Could you check a few things on this model? Use its own coordinates, in mm. A direction names the side the tool comes from. Give positions to 0.01 mm unless a question says otherwise; leave off trailing zeros. Order: outer loops, then holes, each group sorted by start corner. A loop starts at its lowest first (then second) coordinate and runs counter-clockwise, first axis right, second up. Notation, with made-up numbers: M 28,65 L 76,65 A26 ccw 76,83 Z; hole C -30.75,-19.75 d11. An arc over 180 degrees is marked long. Answer in a Markdown table with one row per item. Add a question column.
```python
from build123d import *

# Parameters (mm, degrees)
F0_W     = 101.6
F0_H     = 101.6
F1_DEPTH = 101.6
F2_R     = 76.2
F3_DEPTH = 152.4
F4_W     = 50.8
F4_H     = 50.8
F5_DEPTH = 50.8


with BuildPart() as f1:
    # F0 (on Front) → F1 (new body)
    with BuildSketch(Plane.XZ):
        with Locations((50.8, 50.8)):
            Rectangle(F0_W, F0_H)
    extrude(amount=-F1_DEPTH)

    # F2 (on face) → F3 (join)
    with BuildSketch(Plane.XY.offset(101.6)):
        Circle(F2_R)
    extrude(amount=F3_DEPTH)

    # F4 (on face) → F5 (join)
    with BuildSketch(Plane.XY.offset(101.6)):
        with Locations((76.2, 76.2)):
            Rectangle(F4_W, F4_H)
    extrude(amount=F5_DEPTH)


solid = f1.part
```
1. Suppose I cut it at C-C on z = 221. List the corners of the cut face in (x, y) for me.
2. For faces 1 (the flat face through (0, 50, 50)), 2 (the flat face through (79, 50.8, 127)), 3 (the flat face through (50, 0, 52)), which set-ups out of +Z, -Z, +X, -X, +Y, -Y let a thin tool reach every point of the face, with its end or its side?
3. If I drill on line 1 along Z through (x, y) = (34.5, 77); line 2 along Z through (x, y) = (-17, 28), over which ranges is the centre line in solid material (lowest first)? Write a range as [from, to].
4. Suppose I cut it at B-B on x = -45. List the corners of the cut face in (y, z) for me, plus the area to 3 significant figures.
5. Thinking about a two-plate mould opening in X: for faces 4 (the flat face through (25, 84, 101.6)), 5 (the flat face through (50.8, 79, 127)), 6 (the flat face through (101.6, 50, 58)), 7 (the flat face through (76, 77, 152.4)), which applies, pulls with the +X half, pulls with the -X half, needs draft (parallel to the pull), parting line crosses it, or undercut?
6. Will these pins go through, and if not, where does the flat tip stop? P1, Ø22.5, axis at x = 88, z = 117.5, coming from the -Y side; P2, Ø22.5, axis at y = 78, z = 117.5, coming from the -X side; P3, Ø13.5, axis at x = 24.5, y = 82, coming from the +Z side.
7. Suppose I cut it at A-A on z = 139. List the corners of the cut face in (x, y) for me, plus the area to 3 significant figures.
Findings below:
| question | item | result |
|---|---|---|
| 1 | outline | C 0,0 d152.4 |
| 2 | face 1 | -Z, -X, +Y, -Y |
| 2 | face 2 | +Z, +X |
| 2 | face 3 | -Z, +X, -X, -Y |
| 3 | line 1 | [0, 101.6] |
| 3 | line 2 | [101.6, 254] |
| 4 | outline | M -61.49,101.6 L 61.49,101.6 L 61.49,254 L -61.49,254 Z |
| 4 | area | 18,700 mm2 |
| 5 | face 4 | undercut |
| 5 | face 5 | undercut |
| 5 | face 6 | pulls with the +X half |
| 5 | face 7 | needs draft |
| 6 | P1 | y = 50.8 |
| 6 | P2 | x = -36.75 |
| 6 | P3 | z = 101.6 |
| 7 | outline | M 50.8,56.8 A76.2 ccw long 56.8,50.8 L 101.6,50.8 L 101.6,101.6 L 50.8,101.6 Z |
| 7 | area | 20,800 mm2 |
